```python
from build123d import *

# Parameters (mm, degrees)
F2_SIZE = 1.27


with BuildPart() as f1:
    # F0 (on Front) → F1 (revolve)
    with BuildSketch(Plane.XZ):
        Polygon((2.54, 0), (19.05, 0), (19.05, 12.7), (8.1534, 12.7), (8.1534, 16.51), (2.413, 16.51), (2.413, 24.3586), (0, 24.3586), (0, 16.51), (0, 7.874), (2.54, 7.874), align=None)
    revolve(axis=Axis((0, 0, 12.192), (0, 0, -1)))

    # F2
    f2_edges = [f1.edges().sort_by_distance(p)[0] for p in [
        (-2.413, 0, 24.3586),
    ]]
    chamfer(f2_edges, length=F2_SIZE)


solid = f1.part
```
The model under review builds one solid part; all positions refer to its coordinate system, in mm. A direction names the side the tool comes from. Round coordinates to 2 decimals unless told otherwise and drop trailing zeros. Loops run counter-clockwise (first coordinate to the right, second up) from the corner with the lowest first, then second, coordinate; pieces in that order, holes last. Notation, with made-up numbers: (-7, 70.25) -> (9, 70.25) arc R3 cw to (9, 75.25) -> close; hole circle Ø4 at (55, -9). An arc over 180 degrees is marked (long way). Answer as a JSON object with one key per item and string values. Group by question number.
1) We need section A-A on y = 0. Write out the cut boundary in (x, z), then the cut area to 3 significant figures.
2) For pin 1 Ø2 at (x, z) = (-6, 18) entering from +Y; pin 2 Ø5 at (x, y) = (1, -1) entering from +Z; pin 3 Ø4 at (x, z) = (4, 18) entering from -Y; pin 4 Ø1.5 at (y, z) = (-8.5, 7.5) entering from -X, all flat-tipped, find the tip position at first contact; note any pin that passes through.
3) Mouldability with a two-part tool opening along Y and no side actions: class faces 4 (the face through (-4, 0, 0)), 5 (the face through (0, 0, 7.874)), 6 (the face through (-1.061, -8.084, 14.632)) as released by +Y, released by -Y, zero draft, split by the parting line, or undercut.
4) We need section D-D on z = 7.25. Write out the cut boundary in (x, y), then the cut area to 3 significant figures.
5) For line 1 (X direction, y = 0, z = 4.25); line 2 (Z direction, x = 2, y = 8.5), list the stretches that pass through material, from the lowest coordinate up. Write a range as [from, to].
6) For faces 1 (the face through (8, 4, 12.7)), 2 (the face through (0, 0, 24.359)), 3 (the face through (-0.33, -2.52, 3.88)), list the 3-axis set-ups (+Z, -Z, +X, -X, +Y, -Y) from which the entire face can be reached by the end or side of a thin tool; tool diameter is ignored.
7) We need section C-C on z = 22.5. Write out the cut boundary in (x, y).
Result set:
{
 "1": {"outline": "(-19.05, 0) -> (-2.54, 0) -> (-2.54, 7.87) -> (2.54, 7.87) -> (2.54, 0) -> (19.05, 0) -> (19.05, 12.7) -> (8.15, 12.7) -> (8.15, 16.51) -> (2.41, 16.51) -> (2.41, 23.09) -> (1.14, 24.36) -> (-1.14, 24.36) -> (-2.41, 23.09) -> (-2.41, 16.51) -> (-8.15, 16.51) -> (-8.15, 12.7) -> (-19.05, 12.7) -> close", "area": "542 mm²"},
 "2": {"pin 1": "through", "pin 2": "z = 24.36", "pin 3": "y = -7.71", "pin 4": "x = -17.4"},
 "3": {"face 4": "zero draft", "face 5": "undercut", "face 6": "split by the parting line"},
 "4": {"outline": "circle Ø38.1 at (0, 0); hole circle Ø5.08 at (0, 0)", "area": "1,120 mm²"},
 "5": {"line 1": "[-19.05, -2.54], [2.54, 19.05]", "line 2": "[0, 12.7]"},
 "6": {"face 1": "+Z", "face 2": "+Z, +X, -X, +Y, -Y", "face 3": "-Z"},
 "7": {"outline": "circle Ø4.83 at (0, 0)"}
}
